Autodesk Inventor part; units mm, degrees
ref_plane "YZ Plane" through (0, 0, 0) normal (1, 0, 0) x (0, 1, 0)
ref_plane "XZ Plane" through (0, 0, 0) normal (0, 1, 0) x (-1, 0, 0)
ref_plane "XY Plane" through (0, 0, 0) normal (0, 0, 1) x (1, 0, 0)
sketch "Sketch1" plane through (0, 0, 0) normal (0, 0, 1) x (1, 0, 0)
  line L0 (0, 0) -> (36, 0)
  line L1 (36, 0) -> (36, 50)
  line L2 (36, 50) -> (0, 50)
  line L3 (0, 50) -> (0, 0)
  dimension "d0" = 36
  dimension "d1" = 50
extrude "Extrusion1" add sketch "Sketch1" along normal mid plane 36
sketch "Sketch2" plane through (0, 50, 18) normal (0, 1, 0) x (1, 0, 0)
  line L0 (28.15, 7.85) -> (7.85, 7.85)
  line L1 (7.85, 7.85) -> (7.85, 28.15)
  line L2 (7.85, 28.15) -> (28.15, 28.15)
  line L3 (28.15, 28.15) -> (28.15, 7.85)
  line L4 (28.15, 7.85) -> (7.85, 28.15) construction
  line L5 (7.85, 7.85) -> (28.15, 28.15) construction
  line L6 (0, 36) -> (0, 0)
  point P0 (0, 18)
  point P1 (18, 18)
  point P2 (0, 18)
  dimension "d4" = 18
  dimension "d5" = 20.3
  dimension "d6" = 20.3
extrude "Extrusion2" cut sketch "Sketch2" against normal blind 33
sketch "Sketch3" plane through (0, 0, 18) normal (0, 0, 1) x (1, 0, 0)
  line L0 (0, 50) -> (0, 0)
  line L1 (0, 0) -> (36, 0)
  point P0 (18, 12)
  dimension "d9" = 18
  dimension "d10" = 12
hole "Hole1" at (18, 12, 18) direction (0, 0, -1) diameter 6.2 end through all
sketch "Sketch8" plane through (7.85, 50, -10.15) normal (0, 0, 1) x (1, 0, 0)
  point P0 (-7.85, -50)
sketch "Sketch11" plane through (0, 0, 18) normal (-1, 0, 0) x (0, 0, 1)
  circle A0 centre (-18, 24) radius 2.6
  line L0 (0, 50) -> (0, 0)
  line L1 (-7.85, 17) -> (-28.15, 17)
  point P0 (-18, 0)
  dimension "d41" = 5.2
  dimension "d42" = 18
  dimension "d43" = 7
extrude "Extrusion6" cut sketch "Sketch11" against normal through all
fillet "Fillet1" radius 10 4 edges at (36, 25, 18) (0, 25, 18) (0, 25, -18) (36, 25, -18)
fillet "Fillet2" radius 5 8 edges at (18, 0, 18) (33.0711, 0, 15.0711) (36, 0, 0) (33.0711, 0, -15.0711) (18, 0, -18) (2.9289, 0, -15.0711) (0, 0, 0) (2.9289, 0, 15.0711)
fillet "Fillet3" radius 6.8 8 edges at (33.0711, 50, 15.0711) (18, 50, 18) (2.9289, 50, 15.0711) (0, 50, 0) (2.9289, 50, -15.0711) (18, 50, -18) (33.0711, 50, -15.0711) (36, 50, 0)
properties part number "arm_collar"
Work out the finished part from the listing and answer in its coordinate system (mm). A direction names the side the tool comes from. Coordinates: 2 decimals unless noted, no trailing zeros. Loops run counter-clockwise (first coordinate to the right, second up) from the corner with the lowest first, then second, coordinate; pieces in that order, holes last.
1) For a pull along Y with two mould halves and no side action, classify faces 1 (the cylindrical face through (2.85, 23.83, -14.99)), 2 (the cylindrical face through (3.87, 26.578, -0.338)), 3 (the flat face through (18, 17, 0)) as +Y half, -Y half, draft (parallel to the pull), parting line (faces both ways), or undercut.
Results:
face 1: draft
face 2: undercut
face 3: +Y half
2) Section C-C (x = 18) is taken. Give the vertices of the cut face in (y, z), plus the area to 3 significant figures.
Results:
outline: (0, -13) arc R5 ccw to (5, -18) - (8.9, -18) - (8.9, 18) - (5, 18) arc R5 ccw to (0, 13) - close; (15.1, -18) - (43.2, -18) arc R6.8 ccw to (50, -11.2) - (50, -10.15) - (17, -10.15) - (17, 10.15) - (50, 10.15) - (50, 11.2) arc R6.8 ccw to (43.2, 18) - (15.1, 18) - close
area: 876 mm2
3) Consider probe 1 along Z at (x, y) = (14, 34); probe 2 along X at (y, z) = (33.5, 5.5); probe 3 along Y at (x, z) = (18, 3.5). Determine where each line is inside the solid, lowest interval first.
Results:
probe 1: z = -18 to -10.15, 10.15 to 18
probe 2: x = 0 to 7.85, 28.15 to 36
probe 3: y = 0 to 8.9, 15.1 to 17
4) Section D-D (y = 19) is taken. Give the vertices of the cut face in (x, z).
Results:
outline: (0, -8) arc R10 ccw to (10, -18) - (26, -18) arc R10 ccw to (36, -8) - (36, 8) arc R10 ccw to (26, 18) - (10, 18) arc R10 ccw to (0, 8) - close; hole (7.85, -10.15) - (28.15, -10.15) - (28.15, 10.15) - (7.85, 10.15) - close
5) For faces 4 (the flat face through (18, 24, 18)), 5 (the flat face through (18, 34, -10.15)), determine the directions among +Z, -Z, +X, -X, +Y, -Y from which every point of the face is accessible in a straight line to the end or side of a thin tool.
Results:
face 4: +Z, +X, -X, +Y, -Y
face 5: +Y
6) Section A-A (z = 0) is taken. Give the vertices of the cut face in (x, y).
Results:
outline: (0, 5) arc R5 ccw to (5, 0) - (31, 0) arc R5 ccw to (36, 5) - (36, 21.4) - (28.15, 21.4) - (28.15, 17) - (7.85, 17) - (7.85, 21.4) - (0, 21.4) - close; (0, 26.6) - (7.85, 26.6) - (7.85, 50) - (6.8, 50) arc R6.8 ccw to (0, 43.2) - close; (28.15, 26.6) - (36, 26.6) - (36, 43.2) arc R6.8 ccw to (29.2, 50) - (28.15, 50) - close; hole circle Ø6.2 at (18, 12)
7) Section B-B (y = 12) is taken. Give the vertices of the cut face in (x, z).
Results:
outline: (0, -8) arc R10 ccw to (10, -18) - (14.9, -18) - (14.9, 18) - (10, 18) arc R10 ccw to (0, 8) - close; (21.1, -18) - (26, -18) arc R10 ccw to (36, -8) - (36, 8) arc R10 ccw to (26, 18) - (21.1, 18) - close
8) Flat-ended cylindrical pins translate along their axes: pin 1 (1.5 mm diameter, centred on y = 35, z = 13, fed in from -X); pin 2 (4 mm diameter, centred on y = 34.5, z = -13.5, fed in from -X); pin 3 (4 mm diameter, centred on x = 32, z = 10.5, fed in from +Y). Find the tip coordinate at first contact, or state that the pin passes through.
Results:
pin 1: stops at x = 0.95
pin 2: stops at x = 0.63
pin 3: stops at y = 49.87
